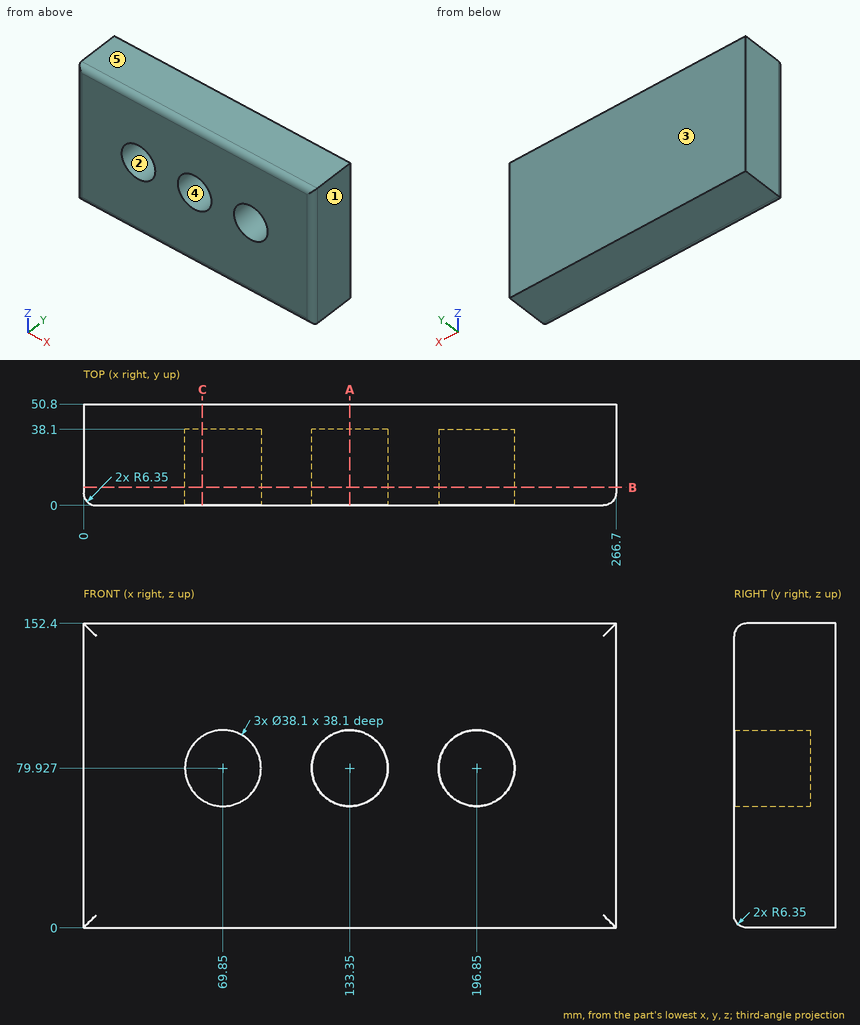
Here's the drawing with two shaded views (mm, measured from the low corner). I have some questions. A direction names the side the tool comes from. Give positions to 0.01 mm unless a question says otherwise; leave off trailing zeros. Write each loop counter-clockwise with the first axis right and the second up, starting at its lowest first coordinate (ties: lowest second). Pieces come first, ordered by that corner, then holes. Notation, with made-up numbers: (18.5, -39.5) -> (62.5, -39.5) arc R17 ccw to (62.5, -13.5) -> close; hole circle Ø2 at (-22, 31). An arc over 180 degrees is marked (long way). Answer as a JSON object with one key per item and string values. Group by question number.
Item 1: Suppose I cut it at C-C (x = 59.5). Please give me the cut outline in (y, z).
Item 2: Please list where these lines run through material, in increasing order: line 1 (Z direction, x = 69, y = 12); line 2 (X direction, y = 3, z = 78.5) (1 decimal); line 3 (X direction, y = 15, z = 95). Write a range as [from, to].
Item 3: We'd pull the mould along X, two halves only. Please class the marked faces 1, 2 and 3: +X half, -X half, draft (parallel to the pull), parting line (faces both ways), or undercut.
Item 4: Suppose I cut it at B-B (y = 9). Please give me the cut outline in (x, z).
Item 5: Suppose I cut it at A-A (x = 133.35). Please give me the cut outline in (y, z).
Item 6: For the marked faces 4 and 5, which set-ups out of +Z, -Z, +X, -X, +Y, -Y let a thin tool reach every point of the face, with its end or its side?
Item 7: I'm going to push a flat-ended pin straight in: P1, Ø19, axis at x = 137, z = 72, coming from the -Y side. Where does the tip first touch, or does it pass through?
Findings:
{
 "1": {"outline": "(0, 6.35) arc R6.35 ccw to (6.35, 0) -> (50.8, 0) -> (50.8, 152.4) -> (6.35, 152.4) arc R6.35 ccw to (0, 146.05) -> (0, 95.92) -> (38.1, 95.92) -> (38.1, 63.93) -> (0, 63.93) -> close"},
 "2": {"line 1": "z = [0, 60.9], [98.96, 152.4]", "line 2": "x = [1, 50.9], [88.8, 114.4], [152.3, 177.9], [215.8, 265.7]", "line 3": "x = [0, 58.2], [81.5, 121.7], [145, 185.2], [208.5, 266.7]"},
 "3": {"face 1": "+X half", "face 2": "undercut", "face 3": "draft"},
 "4": {"outline": "(0, 0) -> (266.7, 0) -> (266.7, 152.4) -> (0, 152.4) -> close; hole circle Ø38.1 at (69.85, 79.93); hole circle Ø38.1 at (133.35, 79.93); hole circle Ø38.1 at (196.85, 79.93)"},
 "5": {"outline": "(0, 6.35) arc R6.35 ccw to (6.35, 0) -> (50.8, 0) -> (50.8, 152.4) -> (6.35, 152.4) arc R6.35 ccw to (0, 146.05) -> (0, 98.98) -> (38.1, 98.98) -> (38.1, 60.88) -> (0, 60.88) -> close"},
 "6": {"face 4": "-Y", "face 5": "+Z, +X, -X, +Y, -Y"},
 "7": {"P1": "stops at y = 38.1"}
}
